Geometry check sheet. Reference: the model listing, model coordinates, mm. Round coordinates to 2 decimals unless told otherwise and drop trailing zeros. Order: outer loops, then holes, each group sorted by start corner. A loop starts at its lowest first (then second) coordinate and runs counter-clockwise, first axis right, second up. Notation, with made-up numbers: (19.5, 28) - (23.5, 28) arc R18 ccw to (23.5, 63) - close; hole circle Ø9 at (-24, 3.25). An arc over 180 degrees is marked (long way). Write each question's results on one line, items separated by ' | '.
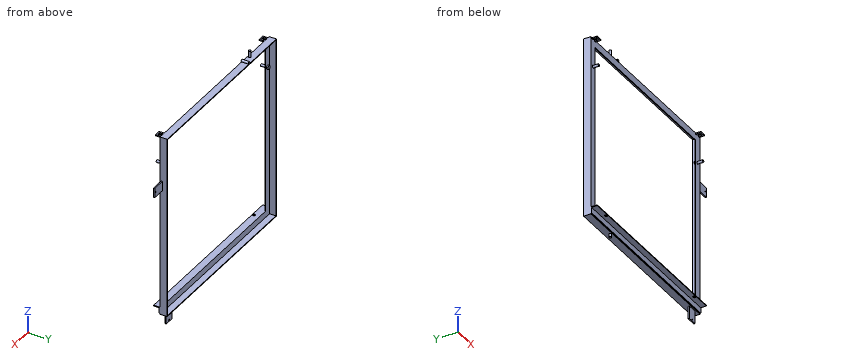
```python
from build123d import *

# Parameters (mm, degrees)
SKETCH_W        = 730.25
SKETCH_H        = 723.9
SKETCH_W_2      = 673.1
SKETCH_H_2      = 666.75
PAD_DEPTH       = 3.175
SKETCH001_W     = 730.25
SKETCH001_H     = 723.9
SKETCH001_W_2   = 723.9
SKETCH001_H_2   = 717.55
PAD001_DEPTH    = 25.4
PAD002_DEPTH    = 730.25
SKETCH003_R     = 5.55625
POCKET_DEPTH    = 28.576
SKETCH004_W     = 23.8125
SKETCH004_H     = 23.8125
SKETCH004_W_2   = 11.1125
SKETCH004_H_2   = 15.875
PAD003_DEPTH    = 4.7625
SKETCH005_R     = 4.7625
PAD004_DEPTH    = 25.4
SKETCH006_R     = 4.7625
PAD005_DEPTH    = 12.7
SKETCH007_R     = 4.826
PAD006_DEPTH    = 28.575
SKETCH008_R     = 5.55625
POCKET001_DEPTH = 28.576
PAD007_DEPTH    = 5.953125
SKETCH010_R     = 4.7625
PAD008_DEPTH    = 25.4
SKETCH011_W     = 38.1
SKETCH011_H     = 4.7625
PAD009_DEPTH    = 50.8
SKETCH012_W     = 38.1
SKETCH012_H     = 4.7625
PAD010_DEPTH    = 50.8
SKETCH013_R     = 2.38125
POCKET002_DEPTH = 28.576


with BuildPart() as part:
    # Sketch → Pad (new body)
    with BuildSketch(Plane.XZ):
        with Locations((365.125, 361.95)):
            Rectangle(SKETCH_W, SKETCH_H)
        with Locations((365.125, 361.95)):
            Rectangle(SKETCH_W_2, SKETCH_H_2, mode=Mode.SUBTRACT)
    extrude(amount=-PAD_DEPTH)

    # Sketch001 (on Face10 of Pad) → Pad001 (join)
    with BuildSketch(Plane(origin=(0, 3.175, 0), x_dir=(1, 0, 0), z_dir=(0, 1, 0))):
        with Locations((365.125, -361.95)):
            Rectangle(SKETCH001_W, SKETCH001_H)
        with Locations((365.125, -361.95)):
            Rectangle(SKETCH001_W_2, SKETCH001_H_2, mode=Mode.SUBTRACT)
    extrude(amount=PAD001_DEPTH)

    # Sketch002 (on Face3 of Pad001) → Pad002 (join)
    with BuildSketch(Plane(origin=(730.25, 0, 0), x_dir=(0, 0, 1), z_dir=(1, 0, 0))):
        Polygon((3.175, 0), (28.575, 0), (28.575, 25.4), (25.4, 25.4), (25.4, 3.175), (3.175, 3.175), align=None)
    extrude(amount=-PAD002_DEPTH)

    # Sketch003 (on Face15 of Pad002) → Pocket (cut, through all)
    with BuildSketch(Plane(origin=(0, 0, 28.575), x_dir=(-1, 0, 0), z_dir=(0, 0, 1))):
        with Locations((-660.4, 19.05)):
            Circle(SKETCH003_R)
        with Locations((-69.85, 19.05)):
            Circle(SKETCH003_R)
    extrude(amount=-POCKET_DEPTH, mode=Mode.SUBTRACT)

    # Sketch004 (on Face6 of Pocket) → Pad003 (join)
    with BuildSketch(Plane(origin=(0, 0, 723.9), x_dir=(-1, 0, 0), z_dir=(0, 0, 1))):
        with Locations((-713.58125, 8.73125)):
            Rectangle(SKETCH004_W, SKETCH004_H)
        with Locations((-713.58125, 7.9375)):
            Rectangle(SKETCH004_W_2, SKETCH004_H_2, mode=Mode.SUBTRACT)
        with Locations((-19.84375, 8.73125)):
            Rectangle(SKETCH004_W, SKETCH004_H)
        with Locations((-19.84375, 7.9375)):
            Rectangle(SKETCH004_W_2, SKETCH004_H_2, mode=Mode.SUBTRACT)
    extrude(amount=-PAD003_DEPTH)

    # Sketch005 (on Face16 of Pad003) → Pad004 (join)
    with BuildSketch(Plane(origin=(0, 0, 723.9), x_dir=(-1, 0, 0), z_dir=(0, 0, 1))):
        with Locations((-142.875, -7.9375)):
            Circle(SKETCH005_R)
    extrude(amount=PAD004_DEPTH)

    # Sketch006 (on Face5 of Pad004) → Pad005 (join)
    with BuildSketch(Plane(origin=(0, 0, 0), x_dir=(1, 0, 0), z_dir=(0, 0, -1))):
        with Locations((142.875, -7.9375)):
            Circle(SKETCH006_R)
    extrude(amount=PAD005_DEPTH)

    # Sketch007 (on Face7 of Pad005) → Pad006 (join)
    with BuildSketch(Plane.XZ):
        with Locations((182.5625, 728.599)):
            Circle(SKETCH007_R)
    extrude(amount=-PAD006_DEPTH)

    # Sketch008 (on Face7 of Pad006) → Pocket001 (cut, through all)
    with BuildSketch(Plane.XZ):
        with Locations((15.875, 609.6)):
            Circle(SKETCH008_R)
        with Locations((714.375, 609.6)):
            Circle(SKETCH008_R)
    extrude(amount=-POCKET001_DEPTH, mode=Mode.SUBTRACT)

    # Sketch009 (on Face49 of Pocket001) → Pad007 (join)
    with BuildSketch(Plane(origin=(0, 3.175, 0), x_dir=(1, 0, 0), z_dir=(0, 1, 0))):
        Polygon((23.01875, -605.475554), (15.875, -601.351108), (8.73125, -605.475554), (8.73125, -613.724446), (15.875, -617.848892), (23.01875, -613.724446), align=None)
        Polygon((714.375, -601.351108), (707.23125, -605.475554), (707.23125, -613.724446), (714.375, -617.848892), (721.51875, -613.724446), (721.51875, -605.475554), align=None)
    extrude(amount=PAD007_DEPTH)

    # Sketch010 (on Face64 of Pad007) → Pad008 (join)
    with BuildSketch(Plane.XZ.offset(-3.175)):
        with Locations((15.875, 609.6)):
            Circle(SKETCH010_R)
        with Locations((714.375, 609.6)):
            Circle(SKETCH010_R)
    extrude(amount=PAD008_DEPTH)

    # Sketch011 (on Face12 of Pad008) → Pad009 (join)
    with BuildSketch(Plane(origin=(730.25, 0, 0), x_dir=(0, 0, 1), z_dir=(1, 0, 0))):
        with Locations((527.05, -7.14375)):
            Rectangle(SKETCH011_W, SKETCH011_H)
    extrude(amount=PAD009_DEPTH)

    # Sketch012 (on Face5 of Pad009) → Pad010 (join)
    with BuildSketch(Plane(origin=(0, 0, 0), x_dir=(1, 0, 0), z_dir=(0, 0, -1))):
        with Locations((685.8, -7.14375)):
            Rectangle(SKETCH012_W, SKETCH012_H)
    extrude(amount=PAD010_DEPTH)

    # Sketch013 (on Face7 of Pad010) → Pocket002 (cut, through all)
    with BuildSketch(Plane.XZ):
        with Locations((774.7, 527.05)):
            Circle(SKETCH013_R)
        with Locations((685.8, -44.45)):
            Circle(SKETCH013_R)
    extrude(amount=-POCKET002_DEPTH, mode=Mode.SUBTRACT)


solid = part.part
```
(1) Section check A-A (x = 352). Record the cut outline in (y, z) (3 decimals).
Answers follow:
outline: (-25.4, 25.4) - (-3.175, 25.4) - (-3.175, 3.175) - (0, 3.175) - (0, 0) - (28.575, 0) - (28.575, 3.175) - (3.175, 3.175) - (3.175, 28.575) - (-25.4, 28.575) - close; (0, 695.325) - (3.175, 695.325) - (3.175, 720.725) - (28.575, 720.725) - (28.575, 723.9) - (0, 723.9) - close
(2) Depth check by flat-ended pin: pin 1 Ø3 at (x, y) = (679.5, 4) entering from -Z; pin 2 Ø23 at (x, y) = (524.5, -13.5) entering from +Z (3 decimals); pin 3 Ø15 at (x, y) = (86.5, -1) entering from +Z; pin 4 Ø4 at (y, z) = (-4.5, 722) entering from -X. Enter the tip coordinate at first touch or a pass-through.
Answers follow:
pin 1: z = -50.8 | pin 2: z = 28.575 | pin 3: z = 723.9 | pin 4: x = 7.94
(3) Material ranges on line 1 (Z direction, x = 685.8, y = 7.05) (3 decimals); line 2 (Z direction, x = 685, y = 8) (3 decimals); line 3 (X direction, y = 8, z = 527) (3 decimals), recorded low to high.
Answers follow:
line 1: -50.8 to -46.831, -42.069 to 3.175, 720.725 to 723.9 | line 2: -50.8 to -46.693, -42.207 to 3.175, 720.725 to 723.9 | line 3: 0 to 3.175, 727.075 to 772.319, 777.081 to 781.05
(4) Section check B-B (z = 574). Record the cut outline in (x, y) (3 decimals).
Answers follow:
outline: (0, 0) - (28.575, 0) - (28.575, 3.175) - (3.175, 3.175) - (3.175, 28.575) - (0, 28.575) - close; (701.675, 0) - (730.25, 0) - (730.25, 28.575) - (727.075, 28.575) - (727.075, 3.175) - (701.675, 3.175) - close
